Job drawing, mm, ordinate dimensions from the low corner. One solid piece. Give positions to 0.01 mm unless a question says otherwise; leave off trailing zeros. Write each loop counter-clockwise with the first axis right and the second up, starting at its lowest first coordinate (ties: lowest second). Pieces come first, ordered by that corner, then holes. Notation, with made-up numbers: M 28,75.5 L 52,75.5 A21 ccw 52,81.5 Z; hole C 67,86 d8. An arc over 180 degrees is marked long. Use CSV: the item, a comma, the result in double quotes. Start each with the question number.
Item 1: Cut at C-C (x = 23). List the corners of the cut face in (y, z), then the cut area to 3 significant figures.
Item 2: Cut at B-B (z = 0.95). List the corners of the cut face in (x, y).
Item 3: Drill centre lines: line 1 (Y direction, x = 23, z = 1); line 2 (X direction, y = 12, z = 0.55). Where is each one in solid material? Low to high. Write a range as [from, to].
Item 4: Cut at A-A (y = 10). List the corners of the cut face in (x, z).
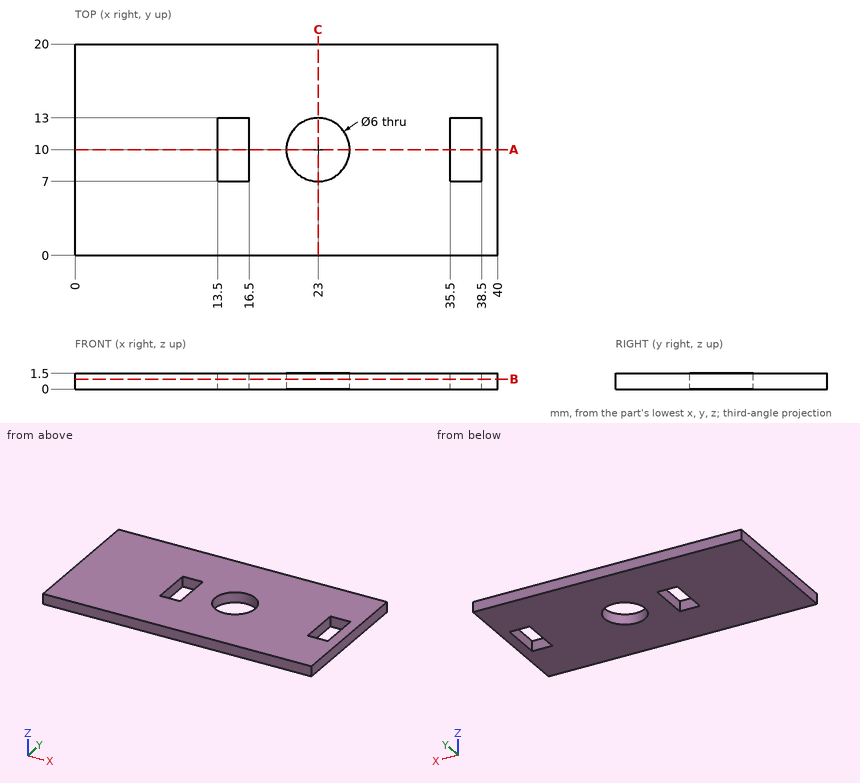
Worked answers:
1,outline,"M 0,0 L 7,0 L 7,1.5 L 0,1.5 Z; M 13,0 L 20,0 L 20,1.5 L 13,1.5 Z"
1,area,"21.0 mm^2"
2,outline,"M 0,0 L 40,0 L 40,20 L 0,20 Z; hole M 13.5,7 L 16.5,7 L 16.5,13 L 13.5,13 Z; hole C 23,10 d6; hole M 35.5,7 L 38.5,7 L 38.5,13 L 35.5,13 Z"
3,line 1,"y = [0, 7], [13, 20]"
3,line 2,"x = [0, 13.5], [16.5, 20.76], [25.24, 35.5], [38.5, 40]"
4,outline,"M 0,0 L 13.5,0 L 13.5,1.5 L 0,1.5 Z; M 16.5,0 L 20,0 L 20,1.5 L 16.5,1.5 Z; M 26,0 L 35.5,0 L 35.5,1.5 L 26,1.5 Z; M 38.5,0 L 40,0 L 40,1.5 L 38.5,1.5 Z"
